```python
from build123d import *

# Parameters (mm, degrees)
F1_DEPTH  = 50.8
F3_DEPTH  = 254.001
F4_W      = 81.28
F4_H      = 76.2
F5_DEPTH  = 50.801
F7_DEPTH  = 177.038
F8_W      = 14.2059672672
F8_H      = 54.5313454777
F8_W_2    = 25.0834482712
F8_H_2    = 56.1428241044
F9_DEPTH  = 50.801
F10_W     = 34.2439590022
F10_H     = 71.3080037385
F11_DEPTH = 50.801
F12_R     = 10.795
F13_DEPTH = 25.4
F14_R     = 10.795
F15_DEPTH = 25.4


# Not quite as in the source:
# - a feature names something its author has since deleted; it is built from what else it names


with BuildPart() as f1:
    # F0 (on Top) → F1 (new body)
    with BuildSketch(Plane.XY):
        Polygon((208.3008480269, 184.2279704243), (-45.6991519731, 184.2279704243), (-45.6991519731, -18.9720295757), (5.1008480269, -69.7720295757), (157.5008480269, -69.7720295757), (208.3008480269, -18.9720295757), align=None)
    extrude(amount=F1_DEPTH)

    # F2 (on face) → F3 (cut, through all)
    with BuildSketch(Plane.YZ.offset(208.3008480269)):
        Polygon((82.6279704243, 50.8), (184.2279704243, 0), (184.2279704243, 50.8), align=None)
    extrude(amount=-F3_DEPTH, mode=Mode.SUBTRACT)

    # F4 (on face) → F5 (cut, through all)
    with BuildSketch(Plane.XY.offset(50.8)):
        with Locations((81.3008480269, -31.6720295757)):
            Rectangle(F4_W, F4_H)
    extrude(amount=-F5_DEPTH, mode=Mode.SUBTRACT)

    # F6 (on face) → F7 (join)
    with BuildSketch(Plane.XZ.offset(69.7720295757)):
        Polygon((-52.88335687, 33.5843649413), (-45.6991519731, 26.4001600444), (-45.6991519731, 40.7685698381), align=None)
        Polygon((208.3008480269, 26.4001600444), (215.4850529237, 33.5843649413), (208.3008480269, 40.7685698381), align=None)
    extrude(amount=-F7_DEPTH)

    # F8 (on face) → F9 (cut, through all)
    with BuildSketch(Plane.XY.offset(50.8)):
        with Locations((-52.8021356067, -46.2377023146)):
            Rectangle(F8_W, F8_H)
        with Locations((220.8425721625, -47.0434416279)):
            Rectangle(F8_W_2, F8_H_2)
    extrude(amount=-F9_DEPTH, mode=Mode.SUBTRACT)

    # F10 (on face) → F11 (cut, through all)
    with BuildSketch(Plane.XY.offset(50.8)):
        with Locations((-2.0932615735, 16.1352222785)):
            Rectangle(F10_W, F10_H)
        with Locations((164.6949576272, 16.1352222785)):
            Rectangle(F10_W, F10_H)
    extrude(amount=-F11_DEPTH, mode=Mode.SUBTRACT)

    # F12 (on face) → F13 (cut)
    with BuildSketch(Plane.YZ.offset(40.6608480269)):
        with Locations((-44.3720295757, 25.4)):
            Circle(F12_R)
    extrude(amount=-F13_DEPTH, mode=Mode.SUBTRACT)

    # F14 (on face) → F15 (cut)
    with BuildSketch(Plane(origin=(121.9408480269, 0, 0), x_dir=(0, -1, 0), z_dir=(-1, 0, 0))):
        with Locations((44.3720295757, 25.4)):
            Circle(F14_R)
    extrude(amount=-F15_DEPTH, mode=Mode.SUBTRACT)


solid = f1.part
```
The listing builds one solid part. Answer for the finished solid, in the listing's coordinates (mm). A direction names the side the tool comes from. Round coordinates to 2 decimals unless told otherwise and drop trailing zeros. Write each loop counter-clockwise with the first axis right and the second up, starting at its lowest first coordinate (ties: lowest second). Pieces come first, ordered by that corner, then holes. Notation, with made-up numbers: (53, 19.5) -> (98, 19.5) arc R25 cw to (98, 31.5) -> close; hole circle Ø8 at (46, 37.25). An arc over 180 degrees is marked (long way). Answer as a JSON object with one key per item and string values. Group by question number.
Q1. Section C-C (z = 11) is taken. Write down the section's boundary in (x, y).
Q2. Which of the six approach directions +Z, -Z, +X, -X, +Y, -Y give full straight-line access (tool end or side, diameter ignored) to faces 1 (the face through (-19.215, 16, 26)), 2 (the face through (-49, -18.972, 34)), 3 (the face through (134.463, -35.805, 18.831)), 4 (the face through (81, 6.428, 26)), 5 (the face through (-49, 107.266, 34))?
Q3. Section D-D (x = 102.5) is taken. Write down the section's boundary in (y, z), plus the area to 3 significant figures.
Q4. Straight lines are drawn through the part: line 1 along X through (y, z) = (20, 47); line 2 along X through (y, z) = (-3, 21); line 3 along Y through (x, z) = (158, 46.5). For each, find the intervals that lie inside material, in ascending order.
Q5. Determine the mould class of faces 6 (the face through (-45.699, 61, 10)), 7 (the face through (23, -69.772, 25)), 8 (the face through (164, 51.789, 26)), 9 (the face through (147.341, -44, 26)) for opening direction X: pulls with the +X half, pulls with the -X half, needs draft (parallel to the pull), parting line crosses it, or undercut.
Q6. Each of these flat-tipped pins is pushed along its axis until it touches: pin 1 Ø5 at (y, z) = (71, 45.5) entering from -X; pin 2 Ø5.5 at (x, z) = (-47.5, 36.5) entering from -Y; pin 3 Ø2 at (x, z) = (148.5, 36) entering from +Y. Where does it stop, or does it pass through?
Q7. Section B-B (x = 36) is taken. Write down the section's boundary in (y, z) (3 decimals).
Q8. Section A-A (y = 45.5) is taken. Write down the section's boundary in (x, z), plus the area to 3 significant figures.
Check values:
{
 "1": {"outline": "(-45.7, -18.97) -> (5.1, -69.77) -> (40.66, -69.77) -> (40.66, 6.43) -> (121.94, 6.43) -> (121.94, -69.77) -> (157.5, -69.77) -> (208.3, -18.97) -> (208.3, 162.23) -> (-45.7, 162.23) -> close; hole (-19.22, -19.52) -> (15.03, -19.52) -> (15.03, 51.79) -> (-19.22, 51.79) -> close; hole (147.57, -19.52) -> (181.82, -19.52) -> (181.82, 51.79) -> (147.57, 51.79) -> close"},
 "2": {"face 1": "+Z, -Z", "face 2": "+Z, -Z, -X, -Y", "face 3": "none", "face 4": "+Z, -Z, -Y", "face 5": "+Z, -Z, -X, +Y"},
 "3": {"outline": "(6.43, 0) -> (184.23, 0) -> (82.63, 50.8) -> (6.43, 50.8) -> close", "area": "6,450 mm^2"},
 "4": {"line 1": "-45.7 to -19.22, 15.03 to 147.57, 181.82 to 208.3", "line 2": "-45.7 to -19.22, 15.03 to 40.66, 121.94 to 147.57, 181.82 to 208.3", "line 3": "-69.27 to -19.52, 51.79 to 91.23"},
 "5": {"face 6": "pulls with the -X half", "face 7": "needs draft", "face 8": "undercut", "face 9": "undercut"},
 "6": {"pin 1": "x = -45.7", "pin 2": "y = -19.92", "pin 3": "y = 114.23"},
 "7": {"outline": "(-69.772, 0) -> (184.228, 0) -> (82.628, 50.8) -> (-69.772, 50.8) -> close; hole circle Ø21.59 at (-44.372, 25.4)"},
 "8": {"outline": "(-52.88, 33.58) -> (-45.7, 26.4) -> (-45.7, 0) -> (-19.22, 0) -> (-19.22, 50.8) -> (-45.7, 50.8) -> (-45.7, 40.77) -> close; (15.03, 0) -> (147.57, 0) -> (147.57, 50.8) -> (15.03, 50.8) -> close; (181.82, 0) -> (208.3, 0) -> (208.3, 26.4) -> (215.49, 33.58) -> (208.3, 40.77) -> (208.3, 50.8) -> (181.82, 50.8) -> close", "area": "9,530 mm^2"}
}
